For this review, take the finished solid that the model builds, in its own axes (mm). A direction names the side the tool comes from. Round coordinates to 2 decimals unless told otherwise and drop trailing zeros. Order: outer loops, then holes, each group sorted by start corner. A loop starts at its lowest first (then second) coordinate and runs counter-clockwise, first axis right, second up. Notation, with made-up numbers: (44, 85) - (63, 85) arc R20 ccw to (63, 107) - close; hole circle Ø11 at (-38, -29). An arc over 180 degrees is marked (long way). One line per question, with ' | ' between items.
```python
from build123d import *

# Parameters (mm, degrees)
EXTRUDE_1_DEPTH          = 25
SKETCH_2_R               = 2.1
CUT_EXTRUDE_1_DEPTH      = 37.249137921
CUT_EXTRUDE_2_DEPTH      = 37.249137921
CUT_EXTRUDE_2_DEPTH_BACK = 37.249137921
SKETCH_2_2_R             = 2.1


with BuildPart() as part:
    # 草图1 → 凸台-拉伸1 (new body)
    with BuildSketch(Plane.XY):
        Polygon((-8, -10), (8, -10), (8, 25), (5, 22), (5, 0), (-5, 0), (-5, 25), (-8, 25), align=None)
    extrude(amount=EXTRUDE_1_DEPTH)

    # 草图2 → 切除-拉伸1 (cut, through all)
    with BuildSketch(Plane(origin=(0, 0, 0), x_dir=(0, 0, -1), z_dir=(1, 0, 0))):
        with Locations((-12.5, 8)):
            Circle(SKETCH_2_R)
        with Locations((-12.5, 18)):
            Circle(SKETCH_2_R)
    extrude(amount=-CUT_EXTRUDE_1_DEPTH, mode=Mode.SUBTRACT)

    # 草图2<2> → 切除-拉伸2 (cut, two sides: drawn at the far end of the back side and taken through both)
    with BuildSketch(Plane(origin=(0, 0, 0), x_dir=(0, 0, -1), z_dir=(1, 0, 0)).offset(-CUT_EXTRUDE_2_DEPTH_BACK)):
        with Locations((-12.5, 8)):
            Circle(SKETCH_2_2_R)
        with Locations((-12.5, 18)):
            Circle(SKETCH_2_2_R)
    extrude(amount=CUT_EXTRUDE_2_DEPTH + CUT_EXTRUDE_2_DEPTH_BACK, mode=Mode.SUBTRACT)


solid = part.part
```
(1) We need section C-C on z = 5. State the section outline as (x, y) points.
Output values:
outline: (-8, -10) - (8, -10) - (8, 25) - (5, 22) - (5, 0) - (-5, 0) - (-5, 25) - (-8, 25) - close
(2) For faces 1 (the cylindrical face through (6.479, 20.082, 12.773)), 2 (the flat face through (5, 11, 12)), list the 3-axis set-ups (+Z, -Z, +X, -X, +Y, -Y) from which the entire face can be reached by the end or side of a thin tool; tool diameter is ignored.
Output values:
face 1: +X, -X | face 2: +Z, -Z, +Y
(3) Mouldability with a two-part tool opening along X and no side actions: class faces 3 (the flat face through (8, 7, 10)), 4 (the flat face through (-5, 12, 12)), 5 (the flat face through (-6, 25, 12)) as released by +X, released by -X, zero draft, split by the parting line, or undercut.
Output values:
face 3: released by +X | face 4: undercut | face 5: zero draft
(4) For probe 1 along Y at (x, z) = (-5.9, 12.5); probe 2 along X at (y, z) = (9.5, 16); probe 3 along Z at (x, y) = (7, 8), list the stretches that pass through material, from the lowest coordinate up. Write a range as [from, to].
Output values:
probe 1: [-10, 5.9], [10.1, 15.9], [20.1, 25] | probe 2: [-8, -5], [5, 8] | probe 3: [0, 10.4], [14.6, 25]
(5) Insertion check: pin 1 (4 mm diameter, centred on x = 5, y = 18.5, fed in from -Z); pin 2 (5 mm diameter, centred on x = 0, z = 10.5, fed in from +Y); pin 3 (2.5 mm diameter, centred on y = 8, z = 12.5, fed in from +X). Each pin has a flat end and moves straight along its axis. Give the tip position at first contact, or say it passes through.
Output values:
pin 1: z = 0 | pin 2: y = 0 | pin 3: through
(6) We need section B-B on z = 12.5. State the section outline as (x, y) points.
Output values:
outline: (-8, -10) - (8, -10) - (8, 5.9) - (5, 5.9) - (5, 0) - (-5, 0) - (-5, 5.9) - (-8, 5.9) - close; (-8, 10.1) - (-5, 10.1) - (-5, 15.9) - (-8, 15.9) - close; (-8, 20.1) - (-5, 20.1) - (-5, 25) - (-8, 25) - close; (5, 10.1) - (8, 10.1) - (8, 15.9) - (5, 15.9) - close; (5, 20.1) - (8, 20.1) - (8, 25) - (5, 22) - close
(7) We need section D-D on y = 9. State the section outline as (x, z) points, plus the area to 3 significant figures.
Output values:
outline: (-8, 0) - (-5, 0) - (-5, 10.65) - (-8, 10.65) - close; (-8, 14.35) - (-5, 14.35) - (-5, 25) - (-8, 25) - close; (5, 0) - (8, 0) - (8, 10.65) - (5, 10.65) - close; (5, 14.35) - (8, 14.35) - (8, 25) - (5, 25) - close | area: 128 mm^2
(8) We need section A-A on y = 18. State the section outline as (x, z) points, plus the area to 3 significant figures.
Output values:
outline: (-8, 0) - (-5, 0) - (-5, 10.4) - (-8, 10.4) - close; (-8, 14.6) - (-5, 14.6) - (-5, 25) - (-8, 25) - close; (5, 0) - (8, 0) - (8, 10.4) - (5, 10.4) - close; (5, 14.6) - (8, 14.6) - (8, 25) - (5, 25) - close | area: 125 mm^2
